Can you work these out from the model? Positions are in its coordinate system, mm. A direction names the side the tool comes from. Coordinates: 2 decimals unless noted, no trailing zeros. Order: outer loops, then holes, each group sorted by start corner. A loop starts at its lowest first (then second) coordinate and runs counter-clockwise, first axis right, second up.
```python
from build123d import *

# Parameters (mm, degrees)
SKETCH1_W               = 228.6
SKETCH1_H               = 228.6
BOSS_EXTRUDE1_DEPTH     = 228.6
CUT_EXTRUDE2_DEPTH      = 396.94681461
CUT_EXTRUDE2_DEPTH_BACK = 396.94681461
SKETCH2_W               = 180.34
SKETCH2_H               = 180.34
SKETCH3_W               = 180.34
SKETCH3_H               = 180.34
CUT_EXTRUDE4_DEPTH      = 396.94681461
SKETCH4_W               = 180.34
SKETCH4_H               = 180.34
CUT_EXTRUDE5_DEPTH      = 396.94681461


with BuildPart() as part:
    # Sketch1 → Boss-Extrude1 (new body)
    with BuildSketch(Plane(origin=(0, 0, 0), x_dir=(1, 0, 0), z_dir=(0, 1, 0))):
        with Locations((114.3, -114.3)):
            Rectangle(SKETCH1_W, SKETCH1_H)
    extrude(amount=BOSS_EXTRUDE1_DEPTH)

    # Sketch2 → Cut-Extrude2 (cut, two sides: drawn at the far end of the back side and taken through both)
    with BuildSketch(Plane.XY.offset(-CUT_EXTRUDE2_DEPTH_BACK)):
        with Locations((114.3, 114.3)):
            Rectangle(SKETCH2_W, SKETCH2_H)
    extrude(amount=CUT_EXTRUDE2_DEPTH + CUT_EXTRUDE2_DEPTH_BACK, mode=Mode.SUBTRACT)

    # Sketch3 → Cut-Extrude4 (cut, through all)
    with BuildSketch(Plane(origin=(0, 0, 0), x_dir=(0, 0, -1), z_dir=(1, 0, 0))):
        with Locations((-114.3, 114.3)):
            Rectangle(SKETCH3_W, SKETCH3_H)
    extrude(amount=CUT_EXTRUDE4_DEPTH, mode=Mode.SUBTRACT)

    # Sketch4 → Cut-Extrude5 (cut, through all)
    with BuildSketch(Plane(origin=(0, 0, 0), x_dir=(1, 0, 0), z_dir=(0, 1, 0))):
        with Locations((114.3, -114.3)):
            Rectangle(SKETCH4_W, SKETCH4_H)
    extrude(amount=CUT_EXTRUDE5_DEPTH, mode=Mode.SUBTRACT)


solid = part.part
```
1. Imagine slicing it at C-C on z = 211. Please give me the cut outline in (x, y), then the cut area to 3 significant figures.
Completed:
outline: (0, 0) - (228.6, 0) - (228.6, 228.6) - (0, 228.6) - close; hole (24.13, 24.13) - (204.47, 24.13) - (204.47, 204.47) - (24.13, 204.47) - close
area: 19,700 mm2
2. Imagine slicing it at A-A on x = 197. Please give me the cut outline in (y, z), then the cut area to 3 significant figures.
Completed:
outline: (0, 0) - (24.13, 0) - (24.13, 24.13) - (0, 24.13) - close; (0, 204.47) - (24.13, 204.47) - (24.13, 228.6) - (0, 228.6) - close; (204.47, 0) - (228.6, 0) - (228.6, 24.13) - (204.47, 24.13) - close; (204.47, 204.47) - (228.6, 204.47) - (228.6, 228.6) - (204.47, 228.6) - close
area: 2,330 mm2
3. On a 3-axis mill with a long thin cutter (end or side, diameter ignored), from which of +Z, -Z, +X, -X, +Y, -Y can I reach the whole of each face in a straight line? I mean faces 1 (the flat face through (113, 204.47, 12)), 2 (the flat face through (11, 113, 228.6)), 3 (the flat face through (0, 113, 218)), 4 (the flat face through (24.13, 12, 116)), 5 (the flat face through (12, 113, 24.13)). Say none if no direction works.
Completed:
face 1: +Z, -Z
face 2: +Z, +X, -X, +Y, -Y
face 3: +Z, -Z, -X, +Y, -Y
face 4: +Y, -Y
face 5: +X, -X
4. Please list where this line runs through material, in increasing order: probe 1 along X at (y, z) = (205.5, 56).
Completed:
probe 1: x = 0 to 24.13, 204.47 to 228.6
5. Thinking about a two-plate mould opening in Z: for faces 6 (the flat face through (24.13, 113, 216)), 7 (the flat face through (204.47, 12, 116)), 8 (the flat face through (11, 113, 0)), which applies, pulls with the +Z half, pulls with the -Z half, needs draft (parallel to the pull), parting line crosses it, or undercut?
Completed:
face 6: needs draft
face 7: undercut
face 8: pulls with the -Z half
